from build123d import *

# Parameters (mm, degrees)
F1_DEPTH = 82.55
F3_D     = 3.81
F5_D     = 3.81


with BuildPart() as f1:
    # F0 (on Top) → F1 (new body)
    with BuildSketch(Plane.XY):
        Polygon((25.4, 25.4), (-25.4, 25.4), (-25.4, -25.4), (-22.225, -25.4), (-22.225, 22.225), (25.4, 22.225), align=None)
    extrude(amount=F1_DEPTH)

    # F3 (through all)
    with Locations(Plane(origin=(-25.4, 0, 0), x_dir=(0, -1, 0), z_dir=(-1, 0, 0))):
        with Locations((12.7, 69.85), (12.7, 44.45)):
            Hole(F3_D / 2)

    # F5 (through all)
    with Locations(Plane(origin=(0, 25.4, 0), x_dir=(-1, 0, 0), z_dir=(0, 1, 0))):
        with Locations((-12.7, 69.85), (-12.7, 44.45)):
            Hole(F5_D / 2)


solid = f1.part
Could you check a few things on this model? Use its own coordinates, in mm. A direction names the side the tool comes from. Give positions to 0.01 mm unless a question says otherwise; leave off trailing zeros. Order: outer loops, then holes, each group sorted by start corner. A loop starts at its lowest first (then second) coordinate and runs counter-clockwise, first axis right, second up.
1. Suppose I cut it at A-A (z = 69.85). List the corners of the cut face in (x, y) for me (3 decimals), plus the area to 3 significant figures.
2. I need wall thicknesses on L1, parallel to Z at x = -23.1, y = -12.7 (3 decimals); L2, parallel to Y at x = -23.75, z = 69.85 (3 decimals); L3, parallel to Y at x = 0.5, z = 54 (3 decimals). Which ranges of each line are inside material? Lowest first, please.
3. Suppose I cut it at B-B (x = 12.7). List the corners of the cut face in (y, z) for me (3 decimals).
4. For faces 1 (the flat face through (-25.4, 0, 41)), 2 (the flat face through (1, 22.225, 41)), which set-ups out of +Z, -Z, +X, -X, +Y, -Y let a thin tool reach every point of the face, with its end or its side?
5. Will these pins go through, and if not, where does the flat tip stop? P1, Ø3, axis at x = 12.7, z = 44.45, coming from the +Y side; P2, Ø6, axis at y = -12.7, z = 44.45, coming from the +X side (3 decimals); P3, Ø5, axis at x = 12.7, z = 69.85, coming from the -Y side (3 decimals).
6. Suppose I cut it at C-C (y = -12.7). List the corners of the cut face in (x, z) for me (3 decimals).
7. Suppose I cut it at D-D (y = -2.5). List the corners of the cut face in (x, z) for me (3 decimals), plus the area to 3 significant figures.
8. We'd pull the mould along X, two halves only. Please class faces 3 (the flat face through (-22.225, -2, 41)), 4 (the cylindrical face through (14.46, 23.79, 43.72)), 5 (the cylindrical face through (12.45, 23.79, 71.74)), 6 (the cylindrical face through (-23.79, -12.95, 71.74)): pulls with the +X half, pulls with the -X half, needs draft (parallel to the pull), parting line crosses it, or undercut.
Solved:
1. outline: (-25.4, -25.4) - (-22.225, -25.4) - (-22.225, -14.605) - (-25.4, -14.605) - close; (-25.4, -10.795) - (-22.225, -10.795) - (-22.225, 22.225) - (10.795, 22.225) - (10.795, 25.4) - (-25.4, 25.4) - close; (14.605, 22.225) - (25.4, 22.225) - (25.4, 25.4) - (14.605, 25.4) - close
1. area: 288 mm2
2. L1: z = 0 to 42.545, 46.355 to 67.945, 71.755 to 82.55
2. L2: y = -25.4 to -14.605, -10.795 to 25.4
2. L3: y = 22.225 to 25.4
3. outline: (22.225, 0) - (25.4, 0) - (25.4, 42.545) - (22.225, 42.545) - close; (22.225, 46.355) - (25.4, 46.355) - (25.4, 67.945) - (22.225, 67.945) - close; (22.225, 71.755) - (25.4, 71.755) - (25.4, 82.55) - (22.225, 82.55) - close
4. face 1: +Z, -Z, -X, +Y, -Y
4. face 2: +Z, -Z, +X, -Y
5. P1: passes through
5. P2: stops at x = -22.225
5. P3: stops at y = 22.225
6. outline: (-25.4, 0) - (-22.225, 0) - (-22.225, 42.545) - (-25.4, 42.545) - close; (-25.4, 46.355) - (-22.225, 46.355) - (-22.225, 67.945) - (-25.4, 67.945) - close; (-25.4, 71.755) - (-22.225, 71.755) - (-22.225, 82.55) - (-25.4, 82.55) - close
7. outline: (-25.4, 0) - (-22.225, 0) - (-22.225, 82.55) - (-25.4, 82.55) - close
7. area: 262 mm2
8. face 3: pulls with the +X half
8. face 4: undercut
8. face 5: undercut
8. face 6: needs draft
